```python
from build123d import *

# Parameters (mm, degrees)
BOSS_EXTRUDE1_DEPTH      = 19
BOSS_EXTRUDE1_DEPTH_BACK = 4
SKETCH2_R                = 3.15
CUT_EXTRUDE1_DEPTH       = 32
SKETCH3_W                = 10.5
SKETCH3_H                = 10.5
CUT_EXTRUDE2_DEPTH       = 24
FILLET1_R                = 4
SKETCH4_W                = 16
SKETCH4_H                = 23
SKETCH4_W_2              = 10.5
SKETCH4_H_2              = 10.5
BOSS_EXTRUDE2_DEPTH      = 15
SKETCH5_W                = 16
SKETCH5_H                = 1.25
SKETCH5_H_2              = 0.25
CUT_EXTRUDE3_DEPTH       = 48


with BuildPart() as part:
    # Sketch1 → Boss-Extrude1 (new body, two sides)
    with BuildSketch(Plane(origin=(0, 0, 0), x_dir=(1, 0, 0), z_dir=(0, 1, 0))) as boss_extrude1_sk:
        with BuildLine():
            Line((0, 0), (0, 16))
            Line((0, 16), (25.005148766, 16))
            ThreePointArc((25.005148766, 16), (29.005148766, 8), (25.005148766, 0))
            Line((25.005148766, 0), (0, 0))
        make_face()
    extrude(amount=BOSS_EXTRUDE1_DEPTH)
    extrude(boss_extrude1_sk.sketch, amount=-BOSS_EXTRUDE1_DEPTH_BACK)

    # Sketch2 → Cut-Extrude1 (cut)
    with BuildSketch(Plane(origin=(0, 19, 0), x_dir=(1, 0, 0), z_dir=(0, 1, 0))):
        with Locations((18.505148766, 8)):
            Circle(SKETCH2_R)
    extrude(amount=-CUT_EXTRUDE1_DEPTH, mode=Mode.SUBTRACT)

    # Sketch3 → Cut-Extrude2 (cut)
    with BuildSketch(Plane.ZY):
        with Locations((-8, 8)):
            Rectangle(SKETCH3_W, SKETCH3_H)
    extrude(amount=-CUT_EXTRUDE2_DEPTH, mode=Mode.SUBTRACT)

    # Fillet1
    fillet1_edges = [part.edges().sort_by_distance(p)[0] for p in [
        (25.005148766, 7.5, -16),
        (25.005148766, 7.5, 0),
    ]]
    fillet(fillet1_edges, radius=FILLET1_R)

    # Sketch4 → Boss-Extrude2 (add)
    with BuildSketch(Plane.ZY):
        with Locations((-8, 7.5)):
            Rectangle(SKETCH4_W, SKETCH4_H)
        with Locations((-8, 8)):
            Rectangle(SKETCH4_W_2, SKETCH4_H_2, mode=Mode.SUBTRACT)
    extrude(amount=BOSS_EXTRUDE2_DEPTH)

    # Sketch5 → Cut-Extrude3 (cut)
    with BuildSketch(Plane.ZY.offset(15)):
        with Locations((-8, -3.375)):
            Rectangle(SKETCH5_W, SKETCH5_H)
        with Locations((-8, 18.875)):
            Rectangle(SKETCH5_W, SKETCH5_H_2)
    extrude(amount=-CUT_EXTRUDE3_DEPTH, mode=Mode.SUBTRACT)


solid = part.part
```
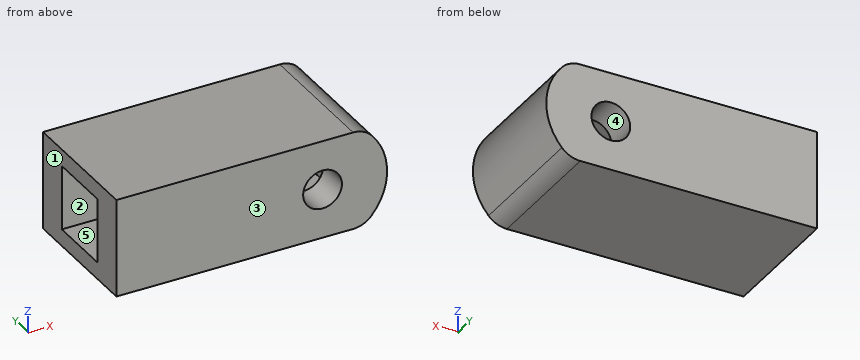
The listing builds one solid part. Answer for the finished solid, in the listing's coordinates (mm). Face numbers are marked on the shaded views. A direction names the side the tool comes from. Coordinates: 2 decimals unless noted, no trailing zeros. Write each loop counter-clockwise with the first axis right and the second up, starting at its lowest first coordinate (ties: lowest second). Pieces come first, ordered by that corner, then holes. Notation, with made-up numbers: M -22.5,39 L -14.5,39 A22 cw -14.5,50 Z; hole C -31,35.5 d9. An arc over 180 degrees is marked long. Use a Markdown table: item, result. Add a question column.
1. Section A-A (z = -8) is taken. Give the vertices of the cut face in (x, y).
2. Section C-C (y = 6.25) is taken. Give the vertices of the cut face in (x, z).
3. For a pull along Y with two mould halves and no side action, classify the marked faces 1, 2 and 3 as +Y half, -Y half, draft (parallel to the pull), parting line (faces both ways), or undercut.
4. Given P1, Ø1, axis at y = 11, z = -6.5, coming from the -X side; P2, Ø4, axis at y = 3.5, z = -12, coming from the +X side, each flat-ended and moving along its own axis, determine where each tip first touches the part or whether it passes through.
5. Section D-D (z = -2) is taken. Give the vertices of the cut face in (x, y).
6. Straight lines are drawn through the part: line 1 along X through (y, z) = (-0.05, -8); line 2 along Z through (x, y) = (5, 8.75); line 3 along Y through (x, z) = (8, -10.25). For each, find the intervals that lie inside material, in ascending order. Write a range as [from, to].
7. Which of the six approach directions +Z, -Z, +X, -X, +Y, -Y give full straight-line access (tool end or side, diameter ignored) to the marked faces 4 and 5?
8. Section B-B (x = 12) is taken. Give the vertices of the cut face in (y, z).
Data:
| question | item | result |
|---|---|---|
| 1 | outline | M -15,-2.75 L 15.36,-2.75 L 15.36,2.75 L -15,2.75 Z; M -15,13.25 L 15.36,13.25 L 15.36,18.75 L -15,18.75 Z; M 21.66,-2.75 L 29.01,-2.75 L 29.01,18.75 L 21.66,18.75 L 21.66,13.25 L 24,13.25 L 24,2.75 L 21.66,2.75 Z |
| 2 | outline | M -15,-16 L 23.48,-16 A4 ccw 26.46,-14.67 A10 ccw 26.46,-1.33 A4 ccw 23.48,0 L -15,0 L -15,-2.75 L 24,-2.75 L 24,-13.25 L -15,-13.25 Z |
| 3 | face 1 | draft |
| 3 | face 2 | undercut |
| 3 | face 3 | -Y half |
| 4 | P1 | stops at x = 24 |
| 4 | P2 | stops at x = 28.8 |
| 5 | outline | M -15,-2.75 L 27.01,-2.75 L 27.01,18.75 L -15,18.75 Z |
| 6 | line 1 | x = [-15, 15.36], [21.66, 29.01] |
| 6 | line 2 | z = [-16, -13.25], [-2.75, 0] |
| 6 | line 3 | y = [-2.75, 2.75], [13.25, 18.75] |
| 7 | face 4 | +Y, -Y |
| 7 | face 5 | -X |
| 8 | outline | M -2.75,-16 L 18.75,-16 L 18.75,0 L -2.75,0 Z; hole M 2.75,-13.25 L 13.25,-13.25 L 13.25,-2.75 L 2.75,-2.75 Z |
